Check sheet for the drawn part. Datum: minimum x, y, z corner. Units: mm. A direction names the side the tool comes from. Give positions to 0.01 mm unless a question says otherwise; leave off trailing zeros. Loops run counter-clockwise (first coordinate to the right, second up) from the corner with the lowest first, then second, coordinate; pieces in that order, holes last.
1. Cross-section at C-C, the plane z = 8. Record the cut outline in (x, y).
2. Tool access check on the marked faces 1 and 2. Record the directions out of +Z, -Z, +X, -X, +Y, -Y that give a thin tool (end or side, any length) a straight path to the whole face; none if there is none.
3. Cross-section at D-D, the plane y = 41.5. Record the cut outline in (x, z), plus the area to 3 significant figures.
4. Go/stop test with flat-tipped pins: pin 1 Ø3.5 at (x, z) = (35.1, 22.5) entering from +Y; pin 2 Ø7 at (x, y) = (14, 24) entering from -Z; pin 3 Ø3 at (y, z) = (25, 17) entering from +X. Record where each tip stops, or that it passes through.
5. Release check for a two-part mould opening along Y. For the marked faces 3 and 4 record: +Y half, -Y half, draft (parallel to the pull), parting line (faces both ways), or undercut.
6. Material ranges on L1, parallel to X at y = 36, z = 22.5; L2, parallel to Y at x = 33.5, z = 7; L3, parallel to X at y = 23.5, z = 41.5, recorded low to high.
7. Cross-section at B-B, the plane x = 39.5. Record the cut outline in (y, z).
8. Cross-section at A-A, the plane x = 26.5. Record the cut outline in (y, z), plus the area to 3 significant figures.
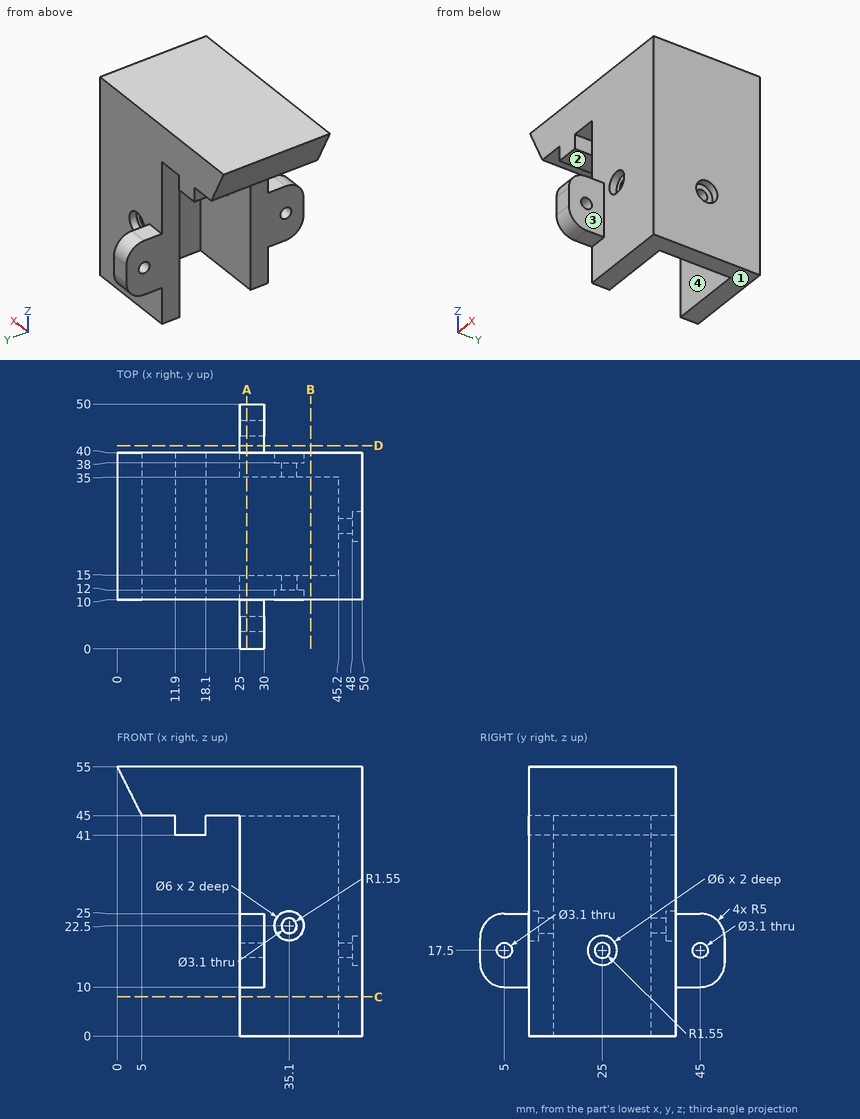
Result:
1. outline: (25, 10) - (50, 10) - (50, 40) - (25, 40) - (25, 35) - (45.2, 35) - (45.2, 15) - (25, 15) - close
2. face 1: -Z, +X, -X, +Y, -Y
2. face 2: -Z, -X, +Y, -Y
3. outline: (25, 10) - (30, 10) - (30, 25) - (25, 25) - close
3. area: 75.0 mm2
4. pin 1: stops at y = 38
4. pin 2: stops at z = 41
4. pin 3: stops at x = 48
5. face 3: draft
5. face 4: undercut
6. L1: x = 25 to 33.55, 36.65 to 50
6. L2: y = 10 to 15, 35 to 40
6. L3: x = 11.9 to 18.1, 45.2 to 50
7. outline: (10, 0) - (15, 0) - (15, 45) - (35, 45) - (35, 0) - (40, 0) - (40, 55) - (10, 55) - close
8. outline: (0, 15) arc R5 ccw to (5, 10) - (10, 10) - (10, 0) - (15, 0) - (15, 45) - (35, 45) - (35, 0) - (40, 0) - (40, 10) - (45, 10) arc R5 ccw to (50, 15) - (50, 20) arc R5 ccw to (45, 25) - (40, 25) - (40, 55) - (10, 55) - (10, 25) - (5, 25) arc R5 ccw to (0, 20) - close; hole circle Ø3.1 at (5, 17.5); hole circle Ø3.1 at (45, 17.5)
8. area: 1,010 mm2
